Geometry check sheet. Reference: the model listing, model coordinates, mm. A direction names the side the tool comes from. Give positions to 0.01 mm unless a question says otherwise; leave off trailing zeros. Write each loop counter-clockwise with the first axis right and the second up, starting at its lowest first coordinate (ties: lowest second). Pieces come first, ordered by that corner, then holes. Notation, with made-up numbers: M 51,-33.75 L 72,-33.75 A29 ccw 72,-9.75 Z; hole C 13,67 d5. An arc over 180 degrees is marked long. One line per item, written item: value. Start each with the question number.
1. Scan lines: line 1 (Z direction, x = 5.5, y = 22); line 2 (X direction, y = 23.5, z = 4.25); line 3 (X direction, y = 22, z = 5.5). Record each from-to range of solid material in increasing order.
2. Cross-section at B-B on z = -0.5. Record the cut outline in (x, y), then the cut area to 3 significant figures.
3. Cross-section at C-C on y = 17.5. Record the cut outline in (x, z) (1 decimal).
4. Gauge pin test, flat ends, axial feed: pin 1 (5 mm diameter, centred on y = 47.5, z = -4, fed in from -X); pin 2 (6 mm diameter, centred on y = 13.5, z = -7.5, fed in from -X); pin 3 (3 mm diameter, centred on x = 15.5, y = 77, fed in from -Z). Record the tip position at first contact, or that the pin passes through.
5. Cross-section at A-A on x = 3.5. Record the cut outline in (y, z) (1 decimal), then the cut area to 3 significant figures.
6. Tool access check on faces 1 (the face through (-0.02, 46.36, -5.61)), 2 (the face through (20, 91.44, 0)), 3 (the face through (-0.486, 45.08, 5.612)). Record the directions out of +Z, -Z, +X, -X, +Y, -Y that give a thin tool (end or side, any length) a straight path to the whole face; none if there is none.
7. Cross-section at D-D on z = -6. Record the cut outline in (x, y), then the cut area to 3 significant figures.
Autodesk Inventor part; units mm, degrees
ref_plane "YZ Plane" through (0, 0, 0) normal (1, 0, 0) x (0, 1, 0)
ref_plane "XZ Plane" through (0, 0, 0) normal (0, 1, 0) x (-1, 0, 0)
ref_plane "XY Plane" through (0, 0, 0) normal (0, 0, 1) x (1, 0, 0)
sketch "Sketch1" plane through (0, 0, 0) normal (0, 0, 1) x (1, 0, 0)
  line L0 (-30.9834, 0) -> (43.9922, 0)
  line L1 (0, -18.288) -> (0, 109.728)
  line L2 (0, 0) -> (33.2814, 91.44)
  line L3 (33.2814, 91.44) -> (13.0089, 91.44)
  line L4 (13.0089, 91.44) -> (-20.2726, 0)
  dimension "d0" = 19.05
  dimension "d10" = 20
  dimension "d11" = 91.44
extrude "Extrusion1" add sketch "Sketch1" along normal mid plane 19.05
sketch "Sketch3" plane through (0, 0, 9.525) normal (0, 0, 1) x (1, 0, 0)
  line L0 (-20.2726, 0) -> (13.0089, 91.44)
  line L1 (0, 0) -> (-20.2726, 0)
  line L2 (33.2814, 91.44) -> (0, 0)
  line L3 (13.0089, 91.44) -> (33.2814, 91.44)
  line L4 (-16.8938, 0) -> (16.3876, 91.44)
  dimension "d7" = 3.175
extrude "Extrusion2" cut sketch "Sketch3" against normal blind 7.9375 contours L4 L3 L2 L1
mirror "Mirror1" about plane through (0, 0, 0) normal (0, 0, 1) of "Extrusion2"
properties part number "brace"
Report:
1. line 1: z = -1.59 to 1.59
1. line 2: x = -11.72 to -8.34
1. line 3: x = -12.27 to -8.89
2. outline: M -20.27,0 L 0,0 L 33.28,91.44 L 13.01,91.44 Z
2. area: 1,850 mm^2
3. outline: M -13.9,-9.5 L -10.5,-9.5 L -10.5,-1.6 L 6.4,-1.6 L 6.4,1.6 L -10.5,1.6 L -10.5,9.5 L -13.9,9.5 Z
4. pin 1: stops at x = -3.89
4. pin 2: stops at x = -16.45
4. pin 3: stops at z = -1.59
5. outline: M 9.6,-1.6 L 56,-1.6 L 56,-9.5 L 65.3,-9.5 L 65.3,9.5 L 56,9.5 L 56,1.6 L 9.6,1.6 Z
5. area: 324 mm^2
6. face 1: -Z, +X, -Y
6. face 2: +Z, -Z, +X, -X, +Y
6. face 3: +Z, +X, -Y
7. outline: M -20.27,0 L -16.89,0 L 16.39,91.44 L 13.01,91.44 Z
7. area: 309 mm^2
